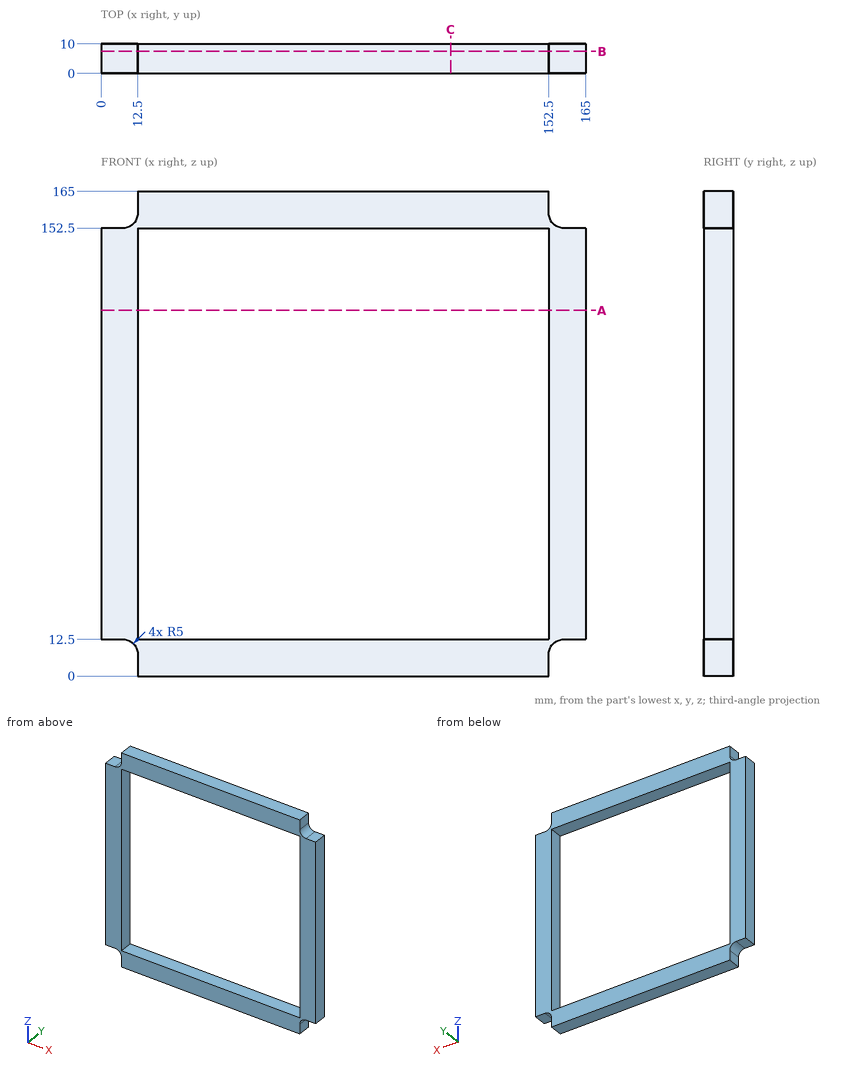
Could you check a few things on this drawing? It's one solid part, dimensions in mm from its lowest x, y, z. Give positions to 0.01 mm unless a question says otherwise; leave off trailing zeros. Order: outer loops, then holes, each group sorted by start corner. A loop starts at its lowest first (then second) coordinate and runs counter-clockwise, first axis right, second up. Notation, with made-up numbers: (10.5, 6.25) - (31.5, 6.25) arc R23 cw to (31.5, 20.25) - close; hole circle Ø6 at (-33.75, 38.5). An arc over 180 degrees is marked (long way). Answer as a JSON object with one key per item and string values. Group by question number.
Item 1: Please list where these lines run through material, in increasing order: probe 1 along X at (y, z) = (1, 55); probe 2 along Z at (x, y) = (8, 7.5).
Item 2: If we section it at B-B on y = 7.5: Please give me the cut outline in (x, z), and give its area (3 significant figures).
Item 3: If we section it at A-A on z = 124.5: Please give me the cut outline in (x, y), and give its area (3 significant figures).
Item 4: For P1, Ø4, axis at y = 6, z = 162.5, coming from the +X side; P2, Ø6, axis at x = 162.5, y = 7, coming from the -Z side; P3, Ø4, axis at y = 4.5, z = 161.5, coming from the -X side, each with a flat end and sliding along its axis, tell me the tip position at first contact or that it passes through.
Item 5: If we section it at C-C on x = 119: Please give me the cut outline in (y, z), and give its area (3 significant figures).
Result set:
{
 "1": {"probe 1": "0 to 12.5, 152.5 to 165", "probe 2": "12.47 to 152.53"},
 "2": {"outline": "(0, 12.5) - (7.5, 12.5) arc R5 cw to (12.5, 7.5) - (12.5, 0) - (152.5, 0) - (152.5, 7.5) arc R5 cw to (157.5, 12.5) - (165, 12.5) - (165, 152.5) - (157.5, 152.5) arc R5 cw to (152.5, 157.5) - (152.5, 165) - (12.5, 165) - (12.5, 157.5) arc R5 cw to (7.5, 152.5) - (0, 152.5) - close; hole (12.5, 12.5) - (152.5, 12.5) - (152.5, 152.5) - (12.5, 152.5) - close", "area": "7,020 mm²"},
 "3": {"outline": "(0, 0) - (12.5, 0) - (12.5, 10) - (0, 10) - close; (152.5, 0) - (165, 0) - (165, 10) - (152.5, 10) - close", "area": "250 mm²"},
 "4": {"P1": "x = 152.5", "P2": "z = 12.5", "P3": "x = 12.5"},
 "5": {"outline": "(0, 0) - (10, 0) - (10, 12.5) - (0, 12.5) - close; (0, 152.5) - (10, 152.5) - (10, 165) - (0, 165) - close", "area": "250 mm²"}
}
